```python
from build123d import *

# Parameters (mm, degrees)
F3_R     = 4
F4_DEPTH = 12
F5_R     = 1.5
F6_DEPTH = 25


with BuildPart() as f1:
    # F0 (on Front) → F1 (revolve)
    with BuildSketch(Plane.XZ):
        with BuildLine():
            Line((0, 19.93), (0, 2.5))
            Line((0, 2.5), (5, 2.5))
            add(Edge.make_bspline(
                [(5, 2.5), (5.3328510826, 2.4217743273), (5.9964782101, 2.2658106511), (6.9983179352, 2.1197039578), (7.9995053084, 2.0366561555), (8.9996417233, 1.9739737746), (9.9999165926, 1.9475438797), (11.0000008446, 1.935865527), (12.0000383829, 1.9489951187), (13.0000622241, 1.9681576208), (14.0000874592, 1.9983838356), (15.0001122592, 2.0383255927), (16.0001370916, 2.0883442574), (17.0001618271, 2.148342783), (18.0001864282, 2.2183478788), (19.0002110875, 2.2983497638), (20.0002349857, 2.3883608236), (21.0002611249, 2.4883412474), (22.0002782257, 2.5984379641), (23.0003283544, 2.7181026114), (24.0002543135, 2.8493833922), (25.000895917, 2.9846630387), (25.9998052646, 3.1525131019), (27.0009227888, 3.3054508496), (28.0009713029, 3.4864375887), (29.0003478858, 3.6897873256), (30.0012434797, 3.8951500576), (31.0002728406, 4.1308468645), (32.0021624026, 4.3625117569), (33.0002529532, 4.6414496195), (34.0023629695, 4.9132136305), (35.0011881909, 5.2289056776), (36.0025557063, 5.5542640629), (37.0014311173, 5.9184670669), (38.0025624421, 6.2958891719), (39.0037946478, 6.7040678184), (40.0028107947, 7.1566870694), (41.0027396353, 7.6374785101), (42.0055454925, 8.1429278876), (43.004228325, 8.7064011364), (44.004224438, 9.306997806), (45.0073247322, 9.9432016714), (46.0057995192, 10.6465378886), (47.0058234103, 11.3970699492), (48.0088937531, 12.1945745949), (49.0086544899, 13.0664036563), (50.0086681154, 14.007093901), (51.009971062, 15.0171879868), (52.0113800481, 16.1070392374), (53.010593298, 17.2897231439), (54.0131863874, 18.5559560931), (54.6684343672, 19.4683264564), (55, 19.93)],
                knots=[0, 0, 0, 0, 0.0192342727, 0.0383486364, 0.0573953442, 0.0764207609, 0.0954333686, 0.1144421761, 0.1334509836, 0.1524612165, 0.1714738242, 0.1904897553, 0.2095099566, 0.2285353734, 0.2475669482, 0.2666056211, 0.285652329, 0.3047080049, 0.3237735783, 0.3428499742, 0.3619381127, 0.3810389089, 0.4001677438, 0.4192965787, 0.4384570424, 0.4576526715, 0.4768671915, 0.4961220706, 0.5153984017, 0.534744074, 0.5541144917, 0.5735639074, 0.5930698576, 0.6126662076, 0.6323264323, 0.6520876645, 0.6719928068, 0.6920124161, 0.7121517577, 0.7325015415, 0.7530286956, 0.7737405025, 0.7947415319, 0.8159934935, 0.837504215, 0.8593884201, 0.8816569315, 0.9043183574, 0.9274369188, 0.9510771906, 0.9752443002, 1, 1, 1, 1], degree=3))
            Line((55, 19.93), (0, 19.93))
        make_face()
    revolve(axis=Axis((0, 0, 5.0231479108), (0, 0, 1)))

    # F3 (on offset) → F4 (join)
    with BuildSketch(Plane.XY.offset(2.8)):
        with Locations((0, -45)):
            Circle(F3_R)
        with Locations((45, 0)):
            Circle(F3_R)
        with Locations((0, 45)):
            Circle(F3_R)
        with Locations((-45, 0)):
            Circle(F3_R)
    extrude(amount=F4_DEPTH)

    # F5 (on offset) → F6 (cut)
    with BuildSketch(Plane.XY.offset(2.8)):
        with Locations((45, 0)):
            Circle(F5_R)
        with Locations((0, -45)):
            Circle(F5_R)
        with Locations((-45, 0)):
            Circle(F5_R)
        with Locations((0, 45)):
            Circle(F5_R)
    extrude(amount=F6_DEPTH, mode=Mode.SUBTRACT)

    # F7 (on Front) → F8 (revolve)
    with BuildSketch(Plane.XZ):
        Polygon((4, 2.5), (0, 2.5), (0, 0.5), align=None)
    revolve(axis=Axis((0, 0, 9.9652772769), (0, 0, 1)))


solid = f1.part
```
Source: CAD feature listing. Evaluate the final solid. Frame: model axes, mm. A direction names the side the tool comes from. Round coordinates to 2 decimals unless told otherwise and drop trailing zeros. Answer as a JSON object with one key per item and string values. Group by question number.
(1) Reachability of faces 1 (the flat face through (-45, -2, 2.8)), 2 (the cylindrical face through (48.815, 1.201, 6.722)), 3 (the flat face through (45, -2, 2.8)), 4 (the flat face through (0, 43, 2.8)) from +Z, -Z, +X, -X, +Y, -Y: full face, straight path, thin tool, end or side. Return the list, or none.
(2) Section query A-A on z = 5. State how many separate pieces and enclosed holes the cut face has, then the cut area to 3 significant figures.
(3) Mould query, pull axis Y, two halves, no side actions, for faces 5 (the cylindrical face through (-49, 0, 7)), 6 (the cylindrical face through (-0.867, -48.905, 6.722)), 7 (the cylindrical face through (-0.521, 48.966, 6.722)), 8 (the flat face through (0, -47, 2.8)). Classes: +Y half, -Y half, draft (parallel to the pull), parting line (faces both ways), or undercut.
(4) First-contact query: pin 1 (1 mm diameter, centred on x = -31.5, z = 12, fed in from +Y); pin 2 (4 mm diameter, centred on x = -36, y = 15.5, fed in from -Z); pin 3 (6.5 mm diameter, centred on x = 45.5, y = 1.5, fed in from -Z). Flat tips, straight axial feed; report the tip coordinate or a pass-through.
(5) Ray query, line 1 (Y direction, x = 0, z = 11.25); line 2 (Y direction, x = -45, z = 10). Return the intervals inside material, ascending. Write a range as [from, to].
Computed values:
{
 "1": {"face 1": "-Z, -X, +Y, -Y", "face 2": "-Z", "face 3": "-Z, +X, +Y, -Y", "face 4": "-Z, +X, -X, +Y"},
 "2": {"separate pieces": "5", "enclosed holes": "4", "area": "3,860 mm^2"},
 "3": {"face 5": "parting line", "face 6": "undercut", "face 7": "undercut", "face 8": "draft"},
 "4": {"pin 1": "y = 36.8", "pin 2": "z = 5.99", "pin 3": "z = 2.8"},
 "5": {"line 1": "[-49, -46.5], [-43.5, 43.5], [46.5, 49]", "line 2": "[-4, -1.5], [1.5, 4]"}
}
